from build123d import *

# Parameters (mm, degrees)
ESQUISSE1_W             = 150
ESQUISSE1_H             = 150
BOSS_EXTRU_1_DEPTH      = 2
CONG_1_R                = 40
BOSS_EXTRU_4_DEPTH      = 2
CONG_2_R                = 40
BOSS_EXTRU_3_DEPTH      = 25.1
ESQUISSE8_R             = 1.45
ENL_V_MAT_EXTRU_4_DEPTH = 8
ENL_V_MAT_EXTRU_6_DEPTH = 42


with BuildPart() as part:
    # Esquisse1 → Boss.-Extru.1 (new body)
    with BuildSketch(Plane.XY):
        Rectangle(ESQUISSE1_W, ESQUISSE1_H)
    extrude(amount=BOSS_EXTRU_1_DEPTH)

    # Congé1
    cong_1_edges = [part.edges().sort_by_distance(p)[0] for p in [
        (-75, 75, 1),
        (75, 75, 1),
        (75, -75, 1),
        (-75, -75, 1),
    ]]
    fillet(cong_1_edges, radius=CONG_1_R)

    # Esquisse9 → Boss.-Extru.4 (add)
    with BuildSketch(Plane.XY.offset(2)):
        with BuildLine():
            Line((35, 75), (100, 75))
            Line((100, 75), (100, -75))
            Line((100, -75), (35, -75))
            ThreePointArc((35, -75), (63.284271247, -63.284271247), (75, -35))
            Line((75, -35), (75, 35))
            ThreePointArc((75, 35), (63.284271247, 63.284271247), (35, 75))
        make_face()
    extrude(amount=-BOSS_EXTRU_4_DEPTH)

    # Congé2
    cong_2_edges = [part.edges().sort_by_distance(p)[0] for p in [
        (100, 75, 1),
        (100, -75, 1),
    ]]
    fillet(cong_2_edges, radius=CONG_2_R)

    # Esquisse5 → Boss.-Extru.3 (add)
    with BuildSketch(Plane(origin=(0, 0, 0), x_dir=(-1, 0, 0), z_dir=(0, 0, -1))):
        with BuildLine():
            Line((-100, 35), (-100, -35))
            ThreePointArc((-100, -35), (-88.284271247, -63.284271247), (-60, -75))
            Line((-60, -75), (35, -75))
            ThreePointArc((35, -75), (63.284271247, -63.284271247), (75, -35))
            Line((75, -35), (75, 35))
            ThreePointArc((75, 35), (63.284271247, 63.284271247), (35, 75))
            Line((35, 75), (-60, 75))
            ThreePointArc((-60, 75), (-88.284271247, 63.284271247), (-100, 35))
        make_face()
        with BuildLine():
            Line((35, 67), (-60, 67))
            ThreePointArc((-60, 67), (-82.627416998, 57.627416998), (-92, 35))
            Line((-92, 35), (-92, -35))
            ThreePointArc((-92, -35), (-82.627416998, -57.627416998), (-60, -67))
            Line((-60, -67), (35, -67))
            ThreePointArc((35, -67), (57.627416998, -57.627416998), (67, -35))
            Line((67, -35), (67, 35))
            ThreePointArc((67, 35), (57.627416998, 57.627416998), (35, 67))
        make_face(mode=Mode.SUBTRACT)
    extrude(amount=BOSS_EXTRU_3_DEPTH)

    # Esquisse8 → Enlèv. mat.-Extru.4 (cut)
    with BuildSketch(Plane(origin=(0, 0, -25.1), x_dir=(-1, 0, 0), z_dir=(0, 0, -1))):
        with Locations((-96, 0)):
            Circle(ESQUISSE8_R)
        with Locations((-12.5, 71)):
            Circle(ESQUISSE8_R)
        with Locations((71, 0)):
            Circle(ESQUISSE8_R)
        with Locations((-12.5, -71)):
            Circle(ESQUISSE8_R)
    extrude(amount=-ENL_V_MAT_EXTRU_4_DEPTH, mode=Mode.SUBTRACT)

    # Esquisse10 → Enlèv. mat.-Extru.6 (cut)
    with BuildSketch(Plane(origin=(100, 0, 0), x_dir=(0, 0, -1), z_dir=(1, 0, 0))):
        with BuildLine():
            Line((0, 10), (0, -10))
            ThreePointArc((0, -10), (10, 0), (0, 10))
        make_face()
    extrude(amount=-ENL_V_MAT_EXTRU_6_DEPTH, mode=Mode.SUBTRACT)


solid = part.part
Geometry check sheet. Reference: the model listing, model coordinates, mm. A direction names the side the tool comes from. Round coordinates to 2 decimals unless told otherwise and drop trailing zeros. Loops run counter-clockwise (first coordinate to the right, second up) from the corner with the lowest first, then second, coordinate; pieces in that order, holes last. Notation, with made-up numbers: (54, -9.5) - (83, -9.5) arc R26 cw to (83, 13.5) - close; hole circle Ø2 at (-26, -18.75). An arc over 180 degrees is marked (long way). One line per question, with ' | ' between items. Start each with the question number.
1. Scan lines: line 1 (Y direction, x = 12.5, z = -22.5); line 2 (Y direction, x = 15.5, z = -17.25); line 3 (X direction, y = 28, z = -11). Record each from-to range of solid material in increasing order. Write a range as [from, to].
2. Depth check by flat-ended pin: pin 1 (1.7 mm diameter, centred on x = 96, y = 0, fed in from -Z); pin 2 (12 mm diameter, centred on y = -49.5, z = -5, fed in from +X). Enter the tip coordinate at first touch or a pass-through.
3. Cross-section at C-C on y = 63. Record the cut outline in (x, z), then the cut area to 3 significant figures.
4. Cross-section at D-D on z = -6.25. Record the cut outline in (x, y).
5. Cross-section at A-A on z = -21.5. Record the cut outline in (x, y), then the cut area to 3 significant figures.
6. Tool access check on faces 4 (the face through (96, 0, -10)), 5 (the face through (14, 1, 2)), 6 (the face through (13, -67, -12)). Record the directions out of +Z, -Z, +X, -X, +Y, -Y that give a thin tool (end or side, any length) a straight path to the whole face; none if there is none.
7. Cross-section at B-B on x = -16.5. Record the cut outline in (y, z).
8. Draft check along Y on faces 1 (the face through (100, 0, -11)), 2 (the face through (92, 0, -12)), 3 (the face through (12, 75, -11)). Enter one of: released by +Y, released by -Y, zero draft, split by the parting line, or undercut.
Taken from the geometry:
1) line 1: [-75, -72.45], [-69.55, -67], [67, 69.55], [72.45, 75] | line 2: [-75, -67], [67, 75] | line 3: [-75, -67], [92, 100]
2) pin 1: z = -17.1 | pin 2: x = 99.09
3) outline: (-63.57, -25.1) - (-50.49, -25.1) - (-50.49, 0) - (75.49, 0) - (75.49, -25.1) - (88.57, -25.1) - (88.57, 2) - (-63.57, 2) - close | area: 961 mm²
4) outline: (-75, -35) arc R40 ccw to (-35, -75) - (60, -75) arc R40 ccw to (100, -35) - (100, -7.81) - (92, -7.81) - (92, -35) arc R32 cw to (60, -67) - (-35, -67) arc R32 cw to (-67, -35) - (-67, 35) arc R32 cw to (-35, 67) - (60, 67) arc R32 cw to (92, 35) - (92, 7.81) - (100, 7.81) - (100, 35) arc R40 ccw to (60, 75) - (-35, 75) arc R40 ccw to (-75, 35) - close
5) outline: (-75, -35) arc R40 ccw to (-35, -75) - (60, -75) arc R40 ccw to (100, -35) - (100, 35) arc R40 ccw to (60, 75) - (-35, 75) arc R40 ccw to (-75, 35) - close; hole circle Ø2.9 at (-71, 0); hole (-67, -35) arc R32 ccw to (-35, -67) - (60, -67) arc R32 ccw to (92, -35) - (92, 35) arc R32 ccw to (60, 67) - (-35, 67) arc R32 ccw to (-67, 35) - close; hole circle Ø2.9 at (12.5, -71); hole circle Ø2.9 at (12.5, 71); hole circle Ø2.9 at (96, 0) | area: 4,420 mm²
6) face 4: +X | face 5: +Z, +X, -X, +Y, -Y | face 6: -Z
7) outline: (-75, -25.1) - (-67, -25.1) - (-67, 0) - (67, 0) - (67, -25.1) - (75, -25.1) - (75, 2) - (-75, 2) - close
8) face 1: zero draft | face 2: undercut | face 3: released by +Y
